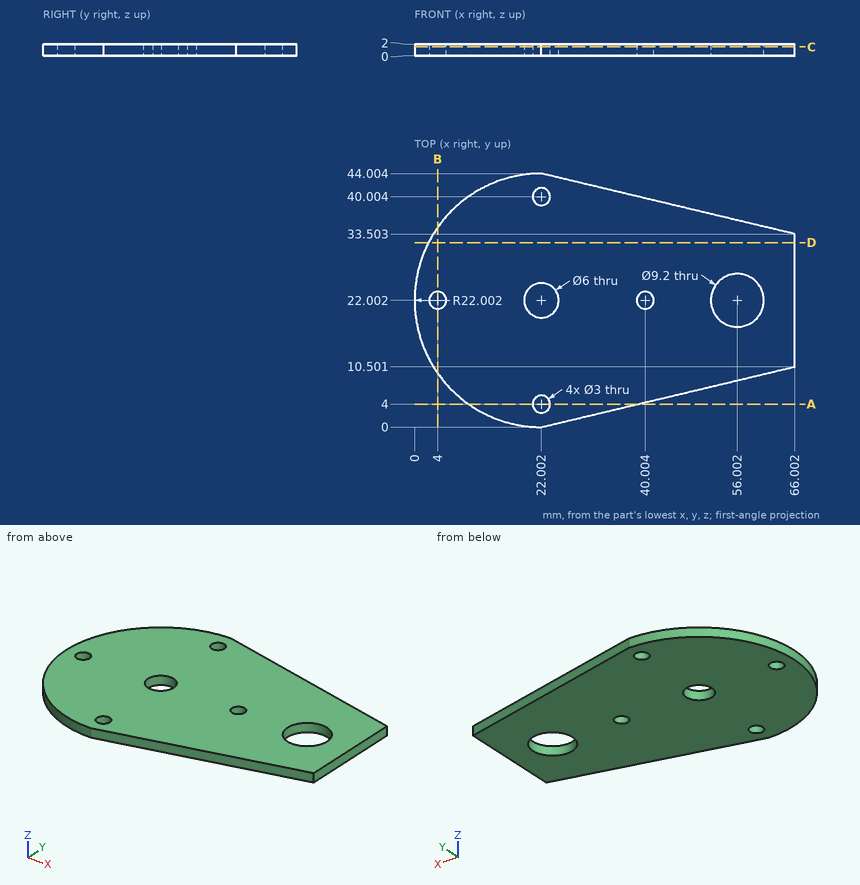
Job drawing, mm, ordinate dimensions from the low corner. One solid piece. Give positions to 0.01 mm unless a question says otherwise; leave off trailing zeros. Loops run counter-clockwise (first coordinate to the right, second up) from the corner with the lowest first, then second, coordinate; pieces in that order, holes last. Notation, with made-up numbers: (31.5, 45.25) -> (89.5, 45.25) arc R29 ccw to (89.5, 78.25) -> close; hole circle Ø3 at (-15.75, 3). An arc over 180 degrees is marked (long way). Use a Markdown table: item, result. Add a question column.
(1) Slice it at D-D on y = 32. List the corners of the cut face in (x, z).
(2) Slice it at B-B on x = 4. List the corners of the cut face in (y, z), and give its area (3 significant figures).
(3) Wall check: line 1 along Y through (x, z) = (59, 0.2); line 2 along Y through (x, z) = (58.5, 1.8); line 3 along X through (y, z) = (30.5, 1.45). Give the ranges that are in metal, low to high.
(4) Slice it at A-A on y = 4. List the corners of the cut face in (x, z), and give its area (3 significant figures).
(5) Slice it at C-C on z = 1.5. List the corners of the cut face in (x, y), and give its area (3 significant figures).
(6) Drop flat-ended pins along their axis: pin 1 Ø12 at (x, y) = (56, 22) entering from -Z; pin 2 Ø2.5 at (x, y) = (22, 4) entering from -Z; pin 3 Ø1 at (y, z) = (11.5, 2) entering from -X. Give the stop position or say it passes through.
Filled sheet:
| question | item | result |
|---|---|---|
| 1 | outline | (2.4, 0) -> (66, 0) -> (66, 2) -> (2.4, 2) -> close |
| 2 | outline | (9.35, 0) -> (20.5, 0) -> (20.5, 2) -> (9.35, 2) -> close; (23.5, 0) -> (34.65, 0) -> (34.65, 2) -> (23.5, 2) -> close |
| 2 | area | 44.6 mm2 |
| 3 | line 1 | 8.83 to 18.51, 25.49 to 35.17 |
| 3 | line 2 | 8.71 to 18.14, 25.86 to 35.29 |
| 3 | line 3 | 1.71 to 66 |
| 4 | outline | (9.35, 0) -> (20.5, 0) -> (20.5, 2) -> (9.35, 2) -> close; (23.5, 0) -> (38.76, 0) -> (38.76, 2) -> (23.5, 2) -> close |
| 4 | area | 52.8 mm2 |
| 5 | outline | (22, 0) -> (66, 10.5) -> (66, 33.5) -> (22, 44) arc R22 ccw to start; hole circle Ø3 at (4, 22); hole circle Ø6 at (22, 22); hole circle Ø3 at (22, 4); hole circle Ø3 at (22, 40); hole circle Ø3 at (40, 22); hole circle Ø9.2 at (56, 22) |
| 5 | area | 2,110 mm2 |
| 6 | pin 1 | z = 0 |
| 6 | pin 2 | through |
| 6 | pin 3 | x = 2.4 |
